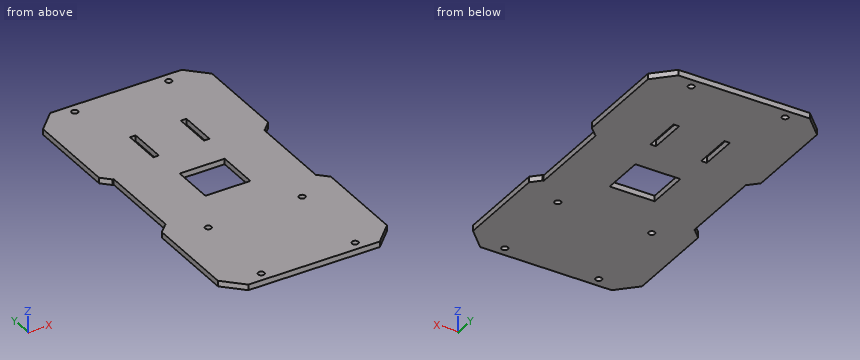
```python
from build123d import *

# Parameters (mm, degrees)
SKETCH1_R           = 1.65
SKETCH1_W           = 3
SKETCH1_H           = 20
SKETCH1_W_2         = 24
SKETCH1_H_2         = 22.230872535
BOSS_EXTRUDE2_DEPTH = 3


with BuildPart() as part:
    # Sketch1 → Boss-Extrude2 (new body)
    with BuildSketch(Plane.XY):
        Polygon((-59.447183423, 47.780041818), (-49.447183423, 57.780041818), (20.552816577, 57.780041818), (30.552816577, 47.780041818), (30.552816577, -0.7691812), (26.052816577, -5.2691812), (25.552816577, -5.2691812), (25.552816577, -50.590735163), (26.052816577, -50.590735163), (30.552816577, -55.090735163), (30.552816577, -103.639958182), (20.552816577, -113.639958182), (-49.447183423, -113.639958182), (-59.447183423, -103.639958182), (-59.447183423, -55.090735163), (-54.947183423, -50.590735163), (-54.447183423, -50.590735163), (-54.447183423, -5.2691812), (-54.947183423, -5.2691812), (-59.447183423, -0.7691812), align=None)
        with Locations((-39.447183423, 52.780041818)):
            Circle(SKETCH1_R, mode=Mode.SUBTRACT)
        with Locations((10.552816577, 52.780041818)):
            Circle(SKETCH1_R, mode=Mode.SUBTRACT)
        with Locations(Location((10.552816577, -108.639958182, 0), (0, 0, 180))):
            Circle(SKETCH1_R, mode=Mode.SUBTRACT)
        with Locations(Location((-39.447183423, -108.639958182, 0), (0, 0, 180))):
            Circle(SKETCH1_R, mode=Mode.SUBTRACT)
        with Locations((10.552816577, -62.748057161)):
            Circle(SKETCH1_R, mode=Mode.SUBTRACT)
        with Locations(Location((-39.447183423, -62.748057161, 0), (0, 0, 180))):
            Circle(SKETCH1_R, mode=Mode.SUBTRACT)
        with Locations((-27.947183423, 11.175041818)):
            Rectangle(SKETCH1_W, SKETCH1_H, mode=Mode.SUBTRACT)
        with Locations((-0.947183423, 11.175041818)):
            Rectangle(SKETCH1_W, SKETCH1_H, mode=Mode.SUBTRACT)
        with Locations((-14.447183423, -27.929958181)):
            Rectangle(SKETCH1_W_2, SKETCH1_H_2, mode=Mode.SUBTRACT)
    extrude(amount=BOSS_EXTRUDE2_DEPTH)


solid = part.part
```
CAD build for the part. Positions are in the model's coordinates, mm. Give positions to 0.01 mm unless a question says otherwise; leave off trailing zeros. Write each loop counter-clockwise with the first axis right and the second up, starting at its lowest first coordinate (ties: lowest second). Pieces come first, ordered by that corner, then holes. Notation, with made-up numbers: (25, 39) -> (57, 39) arc R28 cw to (57, 65) -> close; hole circle Ø4 at (69, 54). An arc over 180 degrees is marked (long way). Write each question's results on one line, items separated by ' | '.
1. Cut at A-A, the plane y = -33. Write the cut outline in (x, z).
Geometry check:
outline: (-54.45, 0) -> (-26.45, 0) -> (-26.45, 3) -> (-54.45, 3) -> close; (-2.45, 0) -> (25.55, 0) -> (25.55, 3) -> (-2.45, 3) -> close
2. Drop flat-ended pins along their axis: P1, Ø1, axis at x = 13.5, y = 18.5, coming from the -Z side; P2, Ø0.6, axis at x = -55, z = 1.5, coming from the -Y side. Give the stop position or say it passes through.
Geometry check:
P1: z = 0 | P2: y = -108.39
3. Cut at B-B, the plane y = 14. Write the cut outline in (x, z).
Geometry check:
outline: (-59.45, 0) -> (-29.45, 0) -> (-29.45, 3) -> (-59.45, 3) -> close; (-26.45, 0) -> (-2.45, 0) -> (-2.45, 3) -> (-26.45, 3) -> close; (0.55, 0) -> (30.55, 0) -> (30.55, 3) -> (0.55, 3) -> close
4. Wall check: probe 1 along Y at (x, z) = (-3, 1.45); probe 2 along Y at (x, z) = (-1.5, 2.75); probe 3 along X at (y, z) = (-18, 0.9). Give the ranges that are in metal, low to high. Write a range as [from, to].
Geometry check:
probe 1: [-113.64, -39.05], [-16.81, 57.78] | probe 2: [-113.64, 1.18], [21.18, 57.78] | probe 3: [-54.45, -26.45], [-2.45, 25.55]
5. Cut at D-D, the plane x = -52. Write the cut outline in (y, z).
Geometry check:
outline: (-111.09, 0) -> (55.23, 0) -> (55.23, 3) -> (-111.09, 3) -> close
6. Cut at C-C, the plane z = 0.7. Give the number of separate pieces and of enclosed holes in the cut face, then the cut area to 3 significant figures.
Geometry check:
separate pieces: 1 | enclosed holes: 9 | area: 14,000 mm²
